Verification items for the finished model (mm, model axes). Coordinates: 2 decimals unless noted, no trailing zeros. Order: outer loops, then holes, each group sorted by start corner. A loop starts at its lowest first (then second) coordinate and runs counter-clockwise, first axis right, second up. Notation, with made-up numbers: M 50.25,56 L 63.25,56 A12 cw 63.25,63 Z; hole C -27,61.5 d8. An arc over 180 degrees is marked long. Return JSON: item names as keys, results as strings.
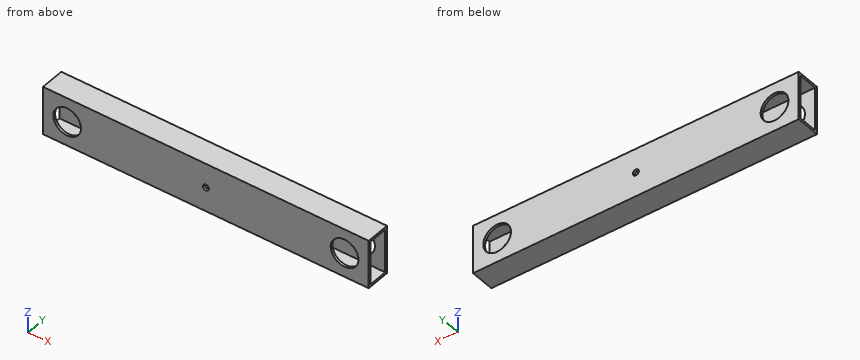
```python
from build123d import *

# Parameters (mm, degrees)
SKETCH1_W           = 50.8
SKETCH1_H           = 25.4
SKETCH1_W_2         = 45.72
SKETCH1_H_2         = 20.32
BOSS_EXTRUDE1_DEPTH = 342.9
SKETCH2_R           = 14.605
CUT_EXTRUDE1_DEPTH  = 345.776347797
SKETCH6_R           = 3.175
CUT_EXTRUDE5_DEPTH  = 345.776347797


with BuildPart() as part:
    # Sketch1 → Boss-Extrude1 (new body)
    with BuildSketch(Plane(origin=(0, 0, 0), x_dir=(0, 0, -1), z_dir=(1, 0, 0))):
        Rectangle(SKETCH1_W, SKETCH1_H)
        Rectangle(SKETCH1_W_2, SKETCH1_H_2, mode=Mode.SUBTRACT)
    extrude(amount=BOSS_EXTRUDE1_DEPTH)

    # Sketch2 → Cut-Extrude1 (cut, through all)
    with BuildSketch(Plane.XZ.offset(12.7)):
        with Locations(Location((25.4, 0, 0), (0, 0, 270))):
            Circle(SKETCH2_R)
        with Locations(Location((317.5, 0, 0), (0, 0, 270))):
            Circle(SKETCH2_R)
    extrude(amount=-CUT_EXTRUDE1_DEPTH, mode=Mode.SUBTRACT)

    # Sketch6 → Cut-Extrude5 (cut, through all)
    with BuildSketch(Plane.XZ.offset(12.7)):
        with Locations(Location((171.45, 0, 0), (0, 0, 270))):
            Circle(SKETCH6_R)
    extrude(amount=-CUT_EXTRUDE5_DEPTH, mode=Mode.SUBTRACT)


solid = part.part
```
Q1. Cross-section at A-A, the plane y = 5.5. Record the boundary of the cut face in (x, z).
Values:
{"outline": "M 0,-25.4 L 342.9,-25.4 L 342.9,-22.86 L 0,-22.86 Z; M 0,22.86 L 342.9,22.86 L 342.9,25.4 L 0,25.4 Z"}
Q2. Cross-section at D-D, the plane x = 251.5. Record the boundary of the cut face in (y, z), and give its area (3 significant figures).
Values:
{"outline": "M -12.7,-25.4 L 12.7,-25.4 L 12.7,25.4 L -12.7,25.4 Z; hole M -10.16,-22.86 L 10.16,-22.86 L 10.16,22.86 L -10.16,22.86 Z", "area": "361 mm^2"}
Q3. Material ranges on line 1 along X through (y, z) = (11.95, 0) (3 decimals); line 2 along Z through (x, y) = (264.5, 3.5); line 3 along Y through (x, z) = (88.5, -17), recorded low to high.
Values:
{"line 1": "0 to 10.795, 40.005 to 168.275, 174.625 to 302.895, 332.105 to 342.9", "line 2": "-25.4 to -22.86, 22.86 to 25.4", "line 3": "-12.7 to -10.16, 10.16 to 12.7"}
Q4. Cross-section at B-B, the plane z = 0. State how many separate pieces and enclosed holes the cut face has, and give its area (3 significant figures).
Values:
{"separate pieces": "8", "enclosed holes": "0", "area": "1,410 mm^2"}
Q5. Cross-section at C-C, the plane x = 25.4. Record the boundary of the cut face in (y, z) (3 decimals).
Values:
{"outline": "M -12.7,-25.4 L 12.7,-25.4 L 12.7,-14.605 L 10.16,-14.605 L 10.16,-22.86 L -10.16,-22.86 L -10.16,-14.605 L -12.7,-14.605 Z; M -12.7,14.605 L -10.16,14.605 L -10.16,22.86 L 10.16,22.86 L 10.16,14.605 L 12.7,14.605 L 12.7,25.4 L -12.7,25.4 Z"}
